from build123d import *

# Parameters (mm, degrees)
BOSS_EXTRUDE1_DEPTH = 1.8
SKETCH2_W           = 6
SKETCH2_H           = 13
BOSS_EXTRUDE2_DEPTH = 0.75
SKETCH7_W           = 6
SKETCH7_H           = 3.8
CUT_EXTRUDE2_DEPTH  = 0.4
SKETCH9_R           = 0.4
CUT_EXTRUDE4_DEPTH  = 0.2
SKETCH10_W          = 4
SKETCH10_H          = 1.1
SKETCH10_H_2        = 3.6
BOSS_EXTRUDE3_DEPTH = 2


with BuildPart() as part:
    # Sketch1 → Boss-Extrude1 (new body)
    with BuildSketch(Plane(origin=(0, 0, 0), x_dir=(1, 0, 0), z_dir=(0, 1, 0))):
        Polygon((-1.4, 3), (-1.4, 0), (-1.975, 0), (-1.975, -1.5), (1.975, -1.5), (1.975, 0), (1.4, 0), (1.4, 3), (3, 3), (3, -10), (-3, -10), (-3, 3), align=None)
    extrude(amount=BOSS_EXTRUDE1_DEPTH)

    # Sketch2 → Boss-Extrude2 (add)
    with BuildSketch(Plane.XZ):
        with Locations((0, 3.5)):
            Rectangle(SKETCH2_W, SKETCH2_H)
    extrude(amount=BOSS_EXTRUDE2_DEPTH)

    # Sketch7 → Cut-Extrude2 (cut)
    with BuildSketch(Plane(origin=(0, 1.8, 0), x_dir=(1, 0, 0), z_dir=(0, 1, 0))):
        with Locations((0, -4.5)):
            Rectangle(SKETCH7_W, SKETCH7_H)
    extrude(amount=-CUT_EXTRUDE2_DEPTH, mode=Mode.SUBTRACT)

    # Sketch9 → Cut-Extrude4 (cut)
    with BuildSketch(Plane(origin=(3, 0, 0), x_dir=(0, 0, -1), z_dir=(1, 0, 0))):
        with Locations((1.9, 0.8)):
            Circle(SKETCH9_R)
    cut_extrude4 = extrude(amount=-CUT_EXTRUDE4_DEPTH, mode=Mode.SUBTRACT)

    # Mirror1: Cut-Extrude4 across plane
    add(cut_extrude4.mirror(Plane(origin=(0, 0, 0), x_dir=(0, 0, 1), z_dir=(1, 0, 0))), mode=Mode.SUBTRACT)

    # Sketch10 → Boss-Extrude3 (add)
    with BuildSketch(Plane(origin=(0, 1.8, 0), x_dir=(1, 0, 0), z_dir=(0, 1, 0))):
        with Locations((0, -2.05)):
            Rectangle(SKETCH10_W, SKETCH10_H)
        with Locations((0, -8.2)):
            Rectangle(SKETCH10_W, SKETCH10_H_2)
    extrude(amount=BOSS_EXTRUDE3_DEPTH)


solid = part.part
Source: CAD feature listing. Evaluate the final solid. Frame: model axes, mm. A direction names the side the tool comes from. Coordinates: 2 decimals unless noted, no trailing zeros. Order: outer loops, then holes, each group sorted by start corner. A loop starts at its lowest first (then second) coordinate and runs counter-clockwise, first axis right, second up.
Item 1: Set-up query: faces 4 (the face through (0, 1.4, 4)), 5 (the face through (2, 3, 2)), 6 (the face through (1.975, 1, 1)), 7 (the face through (1.4, 1, -1)). Return all of +Z, -Z, +X, -X, +Y, -Y with unobstructed straight access to the full face (end or side cutting, diameter ignored); none if empty.
Output values:
face 4: +X, -X, +Y
face 5: +Z, -Z, +X, +Y
face 6: +Y
face 7: -Z, +Y
Item 2: Material intervals for line 1 (Y direction, x = 2.9, z = -1.9); line 2 (Z direction, x = -1.65, y = 0.4); line 3 (Z direction, x = 0.55, y = 3.6), sorted ascending.
Output values:
line 1: y = -0.75 to 0.4, 1.2 to 1.8
line 2: z = -3 to 0, 1.5 to 10
line 3: z = 1.5 to 2.6, 6.4 to 10
Item 3: Cut plane B-B (y = 2.4). Return loops of the section in (x, z).
Output values:
outline: (-2, 1.5) - (2, 1.5) - (2, 2.6) - (-2, 2.6) - close; (-2, 6.4) - (2, 6.4) - (2, 10) - (-2, 10) - close
Item 4: Cut plane D-D (y = 0.8). Return loops of the section in (x, z) (3 decimals), plus the area to 3 significant figures.
Output values:
outline: (-3, -3) - (-1.4, -3) - (-1.4, 0) - (-1.975, 0) - (-1.975, 1.5) - (1.975, 1.5) - (1.975, 0) - (1.4, 0) - (1.4, -3) - (3, -3) - (3, -2.3) - (2.8, -2.3) - (2.8, -1.5) - (3, -1.5) - (3, 10) - (-3, 10) - (-3, -1.5) - (-2.8, -1.5) - (-2.8, -2.3) - (-3, -2.3) - close
area: 63.4 mm2
Item 5: Cut plane C-C (z = -1). Return loops of the section in (x, y).
Output values:
outline: (-3, -0.75) - (3, -0.75) - (3, 1.8) - (1.4, 1.8) - (1.4, 0) - (-1.4, 0) - (-1.4, 1.8) - (-3, 1.8) - close
Item 6: Cut plane A-A (x = 0). Return loops of the section in (y, z).
Output values:
outline: (-0.75, -3) - (0, -3) - (0, 1.5) - (3.8, 1.5) - (3.8, 2.6) - (1.4, 2.6) - (1.4, 6.4) - (3.8, 6.4) - (3.8, 10) - (-0.75, 10) - close
Item 7: First-contact query: P1, Ø0.5, axis at x = 2.5, z = 8, coming from the +Y side; P2, Ø1.9, axis at x = 0, y = 2, coming from the -Z side; P3, Ø1.9, axis at x = -0.5, z = 4, coming from the +Y side; P4, Ø1.5, axis at y = 2, z = 6, coming from the +X side. Flat tips, straight axial feed; report the tip coordinate or a pass-through.
Output values:
P1: stops at y = 1.8
P2: stops at z = 1.5
P3: stops at y = 1.4
P4: stops at x = 3
Item 8: Pull-direction query (Z, two-part tool) for faces 1 (the face through (-1.4, 1, -2)), 2 (the face through (0, -0.3, -3)), 3 (the face through (0, 3, 2.6)); classes: pulls with the +Z half, pulls with the -Z half, needs draft (parallel to the pull), parting line crosses it, or undercut.
Output values:
face 1: needs draft
face 2: pulls with the -Z half
face 3: undercut
